```python
from build123d import *

# Parameters (mm, degrees)
ESBO_O1_W                     = 280
ESBO_O1_H                     = 7.5
ESBO_O3_W                     = 2
ESBO_O3_H                     = 10
RESSALTO_EXTRUS_O1_DEPTH      = 7.5
RESSALTO_EXTRUS_O1_DEPTH_BACK = 7.5
ESBO_O4_W                     = 20
ESBO_O4_H                     = 15
CORTE_EXTRUS_O1_DEPTH         = 7.5
CORTE_EXTRUS_O1_DEPTH_BACK    = 7.5
ESBO_O2_R                     = 2.5


with BuildPart() as part:
    # Esbo_o1 → Revolu_o1 (revolve)
    with BuildSketch(Plane.XY, mode=Mode.PRIVATE) as revolu_o1_sk:
        with Locations((140, -3.75)):
            Rectangle(ESBO_O1_W, ESBO_O1_H)
    revolve(revolu_o1_sk.sketch.rotate(Axis((0, 0, 0), (1, 0, 0)), 270), axis=Axis((0, 0, 0), (1, 0, 0)))

    # Esbo_o3 → Revolu_o2 (revolve)
    with BuildSketch(Plane.XY, mode=Mode.PRIVATE) as revolu_o2_sk:
        with Locations((251, -5)):
            Rectangle(ESBO_O3_W, ESBO_O3_H)
        with Locations((51, -5)):
            Rectangle(ESBO_O3_W, ESBO_O3_H)
    revolve(revolu_o2_sk.sketch.rotate(Axis((50, 0, 0), (1, 0, 0)), 270), axis=Axis((50, 0, 0), (1, 0, 0)))

    # Esbo_o4 → Ressalto-extrus_o1 (add, two sides: drawn at the far end of the back side and taken through both)
    with BuildSketch(Plane.XY.offset(-RESSALTO_EXTRUS_O1_DEPTH_BACK)):
        with Locations((270, 0)):
            Rectangle(ESBO_O4_W, ESBO_O4_H)
    extrude(amount=RESSALTO_EXTRUS_O1_DEPTH + RESSALTO_EXTRUS_O1_DEPTH_BACK)

    # Esbo_o2 → Corte-extrus_o1 (cut, two sides: drawn at the far end of the back side and taken through both)
    with BuildSketch(Plane.XY.offset(-CORTE_EXTRUS_O1_DEPTH_BACK)):
        with Locations((270, 0)):
            Circle(ESBO_O2_R)
    extrude(amount=CORTE_EXTRUS_O1_DEPTH + CORTE_EXTRUS_O1_DEPTH_BACK, mode=Mode.SUBTRACT)


solid = part.part
```
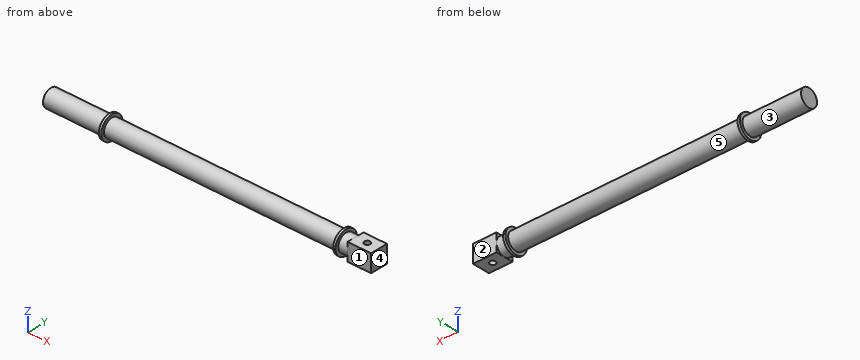
Geometry: final body of the model. Coordinates: model frame, mm. Face numbers are marked on the shaded views. A direction names the side the tool comes from. Round coordinates to 2 decimals unless told otherwise and drop trailing zeros. Loops run counter-clockwise (first coordinate to the right, second up) from the corner with the lowest first, then second, coordinate; pieces in that order, holes last.
Item 1: Section C-C, the plane x = 71. Output: boundary loops of the cut face in (y, z).
Checked values:
outline: circle Ø15 at (0, 0)
Item 2: Contact query for flat-ended pins moving along their axis: P1, Ø6, axis at x = 136, y = 6.5, coming from the -Z side; P2, Ø2, axis at x = 28.5, y = -6.5, coming from the -Z side; P3, Ø4, axis at x = 97.5, z = 4, coming from the +Y side. Output: stop coordinate, or through.
Checked values:
P1: stops at z = -6.63
P2: stops at z = -5.1
P3: stops at y = 7.23
Item 3: Section A-A, the plane x = 270. Output: boundary loops of the cut face in (y, z).
Checked values:
outline: (-7.5, -7.5) - (-2.5, -7.5) - (-2.5, 7.5) - (-7.5, 7.5) - close; (2.5, -7.5) - (7.5, -7.5) - (7.5, 7.5) - (2.5, 7.5) - close
Item 4: Section B-B, the plane z = 2.75. Output: boundary loops of the cut face in (x, y).
Checked values:
outline: (0, -6.98) - (50, -6.98) - (50, -9.61) - (52, -9.61) - (52, -6.98) - (250, -6.98) - (250, -9.61) - (252, -9.61) - (252, -6.98) - (260, -6.98) - (260, -7.5) - (280, -7.5) - (280, 7.5) - (260, 7.5) - (260, 6.98) - (252, 6.98) - (252, 9.61) - (250, 9.61) - (250, 6.98) - (52, 6.98) - (52, 9.61) - (50, 9.61) - (50, 6.98) - (0, 6.98) - close; hole circle Ø5 at (270, 0)
Item 5: Line query: L1, parallel to Y at x = 270, z = -4.5; L2, parallel to X at y = 8, z = -0.25; L3, parallel to Z at x = 152.5, y = -0.5. Output: solid intervals per line, ascending.
Checked values:
L1: y = -7.5 to -2.5, 2.5 to 7.5
L2: x = 50 to 52, 250 to 252
L3: z = -7.48 to 7.48
Item 6: Reachability of the marked faces 1, 2, 3, 4 and 5 from +Z, -Z, +X, -X, +Y, -Y: full face, straight path, thin tool, end or side. Return the list, or none.
Checked values:
face 1: +Z, -Z, +X, -Y
face 2: +Z, -Z, +X, +Y
face 3: -X
face 4: +Z, -Z, +X, +Y, -Y
face 5: none
